Build history of the part. All positions in model axes, mm. A direction names the side the tool comes from. Coordinates: 2 decimals unless noted, no trailing zeros. Order: outer loops, then holes, each group sorted by start corner. A loop starts at its lowest first (then second) coordinate and runs counter-clockwise, first axis right, second up. Notation, with made-up numbers: M 85,30.25 L 118,30.25 A7 cw 118,42.25 Z; hole C -18.75,46 d10. An arc over 180 degrees is marked long. Write item = value, one per line. Start each with the question number.
Q1. Pull direction Z, two halves, no side cores. Call faces 6 (the face through (-27, -2, 0)), 7 (the face through (-31.07, -4.06, -23.5)), 8 (the face through (0, -4, 25)): released by +Z, released by -Z, zero draft, split by the parting line, or undercut.
Q2. Band-saw the part on A-A on y = -1.5. State how many separate pieces and enclosed holes the cut face has, plus the area to 3 significant figures.
Q3. Drill centre lines: probe 1 along Z at (x, y) = (-15.5, -2.1); probe 2 along Z at (x, y) = (-24.5, -7.3); probe 3 along X at (y, z) = (-5.15, -15.5). Where is each one in solid material? Low to high.
Q4. Band-saw the part on B-B on x = -25.5. Write the cut outline in (y, z), plus the area to 3 significant figures.
Q5. Pin check, flat tips, straight feed: P1, Ø6, axis at x = -11.5, z = -17.5, coming from the +Y side; P2, Ø6.5, axis at x = -15.5, z = -15.5, coming from the +Y side; P3, Ø9.5, axis at x = -24.5, z = 15.95, coming from the -Y side; P4, Ø1.9, axis at x = -15.5, z = -15.5, coming from the +Y side. Stop position of each tip, or through.
Q6. 3-axis set-ups, long thin cutter, end or side, ignore diameter. For faces 1 (the face through (-22, -6, -18)), 2 (the face through (27, -2, 0)), 3 (the face through (-31.07, -4.06, 23.5)), 4 (the face through (0, 0, 0)), 5 (the face through (-18.84, -1.92, 16.55)): which of +Z, -Z, +X, -X, +Y, -Y reach the whole face in a straight line?
```python
from build123d import *

# Parameters (mm, degrees)
F0_W     = 65
F0_H     = 50
F0_W_2   = 45
F0_H_2   = 6.7
F1_DEPTH = 8
F2_R     = 6
F2_R_2   = 3.6
F2_R_3   = 5
F2_R_4   = 2.55
F3_DEPTH = 2
F4_W     = 5.5
F4_H     = 6.7
F5_DEPTH = 3
F7_DEPTH = 7
F8_R     = 3.5
F9_DEPTH = 3.9
F10_R    = 5


with BuildPart() as f1:
    # F0 (on Front) → F1 (new body)
    with BuildSketch(Plane.XZ):
        Rectangle(F0_W, F0_H)
        with BuildLine():
            ThreePointArc((-24.5, 12.35), (-27.0455844123, 18.4955844123), (-20.9, 15.95))
            Line((-20.9, 15.95), (20.9, 15.95))
            ThreePointArc((20.9, 15.95), (24.5, 19.55), (28.1, 15.95))
            ThreePointArc((28.1, 15.95), (27.0455844123, 13.4044155877), (24.5, 12.35))
            Line((24.5, 12.35), (24.5, 3.35))
            Line((24.5, 3.35), (27, 3.35))
            Line((27, 3.35), (27, -3.35))
            Line((27, -3.35), (24.5, -3.35))
            Line((24.5, -3.35), (24.5, -13.4))
            ThreePointArc((24.5, -13.4), (26.303122292, -14.146877708), (27.05, -15.95))
            ThreePointArc((27.05, -15.95), (24.5, -18.5), (21.95, -15.95))
            Line((21.95, -15.95), (-21.95, -15.95))
            ThreePointArc((-21.95, -15.95), (-26.303122292, -17.753122292), (-24.5, -13.4))
            Line((-24.5, -13.4), (-24.5, -3.35))
            Line((-24.5, -3.35), (-27, -3.35))
            Line((-27, -3.35), (-27, 3.35))
            Line((-27, 3.35), (-24.5, 3.35))
            Line((-24.5, 3.35), (-24.5, 12.35))
        make_face(mode=Mode.SUBTRACT)
        with BuildLine():
            Line((20.9, 15.95), (-20.9, 15.95))
            ThreePointArc((-20.9, 15.95), (-21.9544155877, 13.4044155877), (-24.5, 12.35))
            Line((-24.5, 12.35), (-24.5, 3.35))
            Line((-24.5, 3.35), (-22.5, 3.35))
            Line((-22.5, 3.35), (22.5, 3.35))
            Line((22.5, 3.35), (24.5, 3.35))
            Line((24.5, 3.35), (24.5, 12.35))
            ThreePointArc((24.5, 12.35), (21.9544155877, 13.4044155877), (20.9, 15.95))
        make_face()
        with BuildLine():
            Line((-22.5, -3.35), (-24.5, -3.35))
            Line((-24.5, -3.35), (-24.5, -13.4))
            ThreePointArc((-24.5, -13.4), (-22.696877708, -14.146877708), (-21.95, -15.95))
            Line((-21.95, -15.95), (21.95, -15.95))
            ThreePointArc((21.95, -15.95), (22.696877708, -14.146877708), (24.5, -13.4))
            Line((24.5, -13.4), (24.5, -3.35))
            Line((24.5, -3.35), (22.5, -3.35))
            Line((22.5, -3.35), (-22.5, -3.35))
        make_face()
        Rectangle(F0_W_2, F0_H_2)
    extrude(amount=F1_DEPTH)

    # F2 (on face) → F3 (cut)
    with BuildSketch(Plane.XZ.offset(8)):
        with Locations((24.5, 15.95)):
            Circle(F2_R)
        with Locations((24.5, 15.95)):
            Circle(F2_R_2, mode=Mode.SUBTRACT)
        with Locations((-24.5, 15.95)):
            Circle(F2_R)
        with Locations((-24.5, 15.95)):
            Circle(F2_R_2, mode=Mode.SUBTRACT)
        with Locations((-24.5, -15.95)):
            Circle(F2_R_3)
        with Locations((-24.5, -15.95)):
            Circle(F2_R_4, mode=Mode.SUBTRACT)
        with Locations((24.5, -15.95)):
            Circle(F2_R_3)
        with Locations((24.5, -15.95)):
            Circle(F2_R_4, mode=Mode.SUBTRACT)
    extrude(amount=-F3_DEPTH, mode=Mode.SUBTRACT)

    # F4 (on face) → F5 (cut)
    with BuildSketch(Plane.XZ.offset(8)):
        with Locations((29.75, 0)):
            Rectangle(F4_W, F4_H)
        with Locations((-29.75, 0)):
            Rectangle(F4_W, F4_H)
    extrude(amount=-F5_DEPTH, mode=Mode.SUBTRACT)

    # F6 (on face) → F7 (cut)
    with BuildSketch(Plane.XZ.offset(8)):
        with BuildLine():
            Line((-15.5, 17.05), (-15.5, 15.5))
            Line((-15.5, 15.5), (-13.95, 15.5))
            ThreePointArc((-13.95, 15.5), (-14.4039844892, 16.5960155108), (-15.5, 17.05))
        make_face()
        with BuildLine():
            Line((-13.95, 15.5), (-15.5, 15.5))
            Line((-15.5, 15.5), (-15.5, 13.95))
            ThreePointArc((-15.5, 13.95), (-14.4039844892, 14.4039844892), (-13.95, 15.5))
        make_face()
        with BuildLine():
            ThreePointArc((17.05, 15.5), (15.5, 17.05), (13.95, 15.5))
            Line((13.95, 15.5), (15.5, 15.5))
            Line((15.5, 15.5), (15.5, 13.95))
            ThreePointArc((15.5, 13.95), (16.5960155108, 14.4039844892), (17.05, 15.5))
        make_face()
        with BuildLine():
            Line((15.5, 15.5), (13.95, 15.5))
            ThreePointArc((13.95, 15.5), (14.4039844892, 14.4039844892), (15.5, 13.95))
            Line((15.5, 13.95), (15.5, 15.5))
        make_face()
        with BuildLine():
            Line((-15.5, -15.5), (-15.5, -13.95))
            ThreePointArc((-15.5, -13.95), (-16.5960155108, -16.5960155108), (-13.95, -15.5))
            Line((-13.95, -15.5), (-15.5, -15.5))
        make_face()
        with BuildLine():
            ThreePointArc((-13.95, -15.5), (-14.4039844892, -14.4039844892), (-15.5, -13.95))
            Line((-15.5, -13.95), (-15.5, -15.5))
            Line((-15.5, -15.5), (-13.95, -15.5))
        make_face()
        with BuildLine():
            Line((15.5, -15.5), (15.5, -13.95))
            ThreePointArc((15.5, -13.95), (14.4039844892, -14.4039844892), (13.95, -15.5))
            Line((13.95, -15.5), (15.5, -15.5))
        make_face()
        with BuildLine():
            ThreePointArc((17.05, -15.5), (16.5960155108, -14.4039844892), (15.5, -13.95))
            Line((15.5, -13.95), (15.5, -15.5))
            Line((15.5, -15.5), (13.95, -15.5))
            ThreePointArc((13.95, -15.5), (15.5, -17.05), (17.05, -15.5))
        make_face()
        with BuildLine():
            Line((-15.5, 13.95), (-15.5, 15.5))
            Line((-15.5, 15.5), (-15.5, 17.05))
            ThreePointArc((-15.5, 17.05), (-17.05, 15.5), (-15.5, 13.95))
        make_face()
    extrude(amount=-F7_DEPTH, mode=Mode.SUBTRACT)

    # F8 (on face) → F9 (cut)
    with BuildSketch(Plane(origin=(0, 0, 0), x_dir=(-1, 0, 0), z_dir=(0, 1, 0))):
        with Locations((-15.5, 15.5)):
            Circle(F8_R)
        with Locations((-15.5, -15.5)):
            Circle(F8_R)
        with Locations((15.5, 15.5)):
            Circle(F8_R)
        with Locations((15.5, -15.5)):
            Circle(F8_R)
    extrude(amount=-F9_DEPTH, mode=Mode.SUBTRACT)

    # F10
    f10_edges = [f1.edges().sort_by_distance(p)[0] for p in [
        (32.5, -4, 25),
        (32.5, -4, -25),
        (-32.5, -4, 25),
        (-32.5, -4, -25),
    ]]
    fillet(f10_edges, radius=F10_R)


solid = f1.part
```
Recorded:
q1.face_6 = undercut
q1.face_7 = released by -Z
q1.face_8 = released by +Z
q2.separate_pieces = 1
q2.enclosed_holes = 10
q2.area = 2,890 mm2
q3.probe_1 = -25 to -19, -12 to 12, 19 to 25
q3.probe_2 = -25 to -20.95, -10.95 to -3.35, 3.35 to 9.95, 21.95 to 25
q3.probe_3 = -32.5 to -27.01, -21.99 to -17.05, -13.95 to 13.95, 17.05 to 21.99, 27.01 to 32.5
q4.outline = M -8,-25 L 0,-25 L 0,-18.3 L -6,-18.3 L -6,-20.85 L -8,-20.85 Z; M -8,-11.05 L -6,-11.05 L -6,-13.6 L 0,-13.6 L 0,-3.35 L -8,-3.35 Z; M -8,3.35 L 0,3.35 L 0,12.49 L -6,12.49 L -6,10.03 L -8,10.03 Z; M -8,21.87 L -6,21.87 L -6,19.41 L 0,19.41 L 0,25 L -8,25 Z
q4.area = 233 mm2
q5.P1 = 0
q5.P2 = -3.9
q5.P3 = -6
q5.P4 = through
q6.face_1 = -Y
q6.face_2 = +Y, -Y
q6.face_3 = +Z, -X, +Y, -Y
q6.face_4 = +Z, -Z, +X, -X, +Y
q6.face_5 = +Y
